Read the model definition and answer for the solid it produces. Units are mm, in the model's axes. Coordinates: 2 decimals unless noted, no trailing zeros. Write each loop counter-clockwise with the first axis right and the second up, starting at its lowest first coordinate (ties: lowest second). Pieces come first, ordered by that corner, then holes.
Autodesk Inventor part; units mm, degrees
ref_plane "YZ Plane" through (0, 0, 0) normal (1, 0, 0) x (0, 1, 0)
ref_plane "XZ Plane" through (0, 0, 0) normal (0, 1, 0) x (-1, 0, 0)
ref_plane "XY Plane" through (0, 0, 0) normal (0, 0, 1) x (1, 0, 0)
sketch "Sketch1" plane through (0, 0, 0) normal (0, 0, 1) x (1, 0, 0)
  circle A0 centre (0, 0) radius 1.6
  line L0 (-3.75, -3.75) -> (3.75, -3.75)
  line L1 (3.75, -3.75) -> (3.75, 3.75)
  line L2 (3.75, 3.75) -> (-3.75, 3.75)
  line L3 (-3.75, 3.75) -> (-3.75, -3.75)
  point P0 (3.75, 0)
  point P1 (0, 3.75)
  dimension "d0" = 3.2
  dimension "d1" = 7.5
  dimension "d2" = 7.5
extrude "Extrusion1" add sketch "Sketch1" along normal blind 5
chamfer "Chamfer1" distance 1 angle 45 4 edges at (3.75, -3.75, 2.5) (-3.75, -3.75, 2.5) (-3.75, 3.75, 2.5) (3.75, 3.75, 2.5)
properties part number "EndEffector_holder_Touch"
Item 1: The part is cut by section C-C (z = 2.95). Give the vertices of the cut face in (x, y).
Item 2: The part is cut by section A-A (y = 0). Give the vertices of the cut face in (x, z), and give its area (3 significant figures).
Item 3: Given pin 1 (2 mm diameter, centred on x = -1, y = -1, fed in from +Z), flat-ended and moving along its own axis, determine where the tip first touches the part or whether it passes through.
Item 4: Find the intervals of material crossed by probe 1 along Y at (x, z) = (0, 2.25); probe 2 along X at (y, z) = (0.5, 2.3), in increasing order.
Item 5: The part is cut by section D-D (y = 3.5). Give the vertices of the cut face in (x, z).
Answer:
1. outline: (-3.75, -2.75) - (-2.75, -3.75) - (2.75, -3.75) - (3.75, -2.75) - (3.75, 2.75) - (2.75, 3.75) - (-2.75, 3.75) - (-3.75, 2.75) - close; hole circle Ø3.2 at (0, 0)
2. outline: (-3.75, 0) - (-1.6, 0) - (-1.6, 5) - (-3.75, 5) - close; (1.6, 0) - (3.75, 0) - (3.75, 5) - (1.6, 5) - close
2. area: 21.5 mm2
3. pin 1: stops at z = 5
4. probe 1: y = -3.75 to -1.6, 1.6 to 3.75
4. probe 2: x = -3.75 to -1.52, 1.52 to 3.75
5. outline: (-3, 0) - (3, 0) - (3, 5) - (-3, 5) - close
